Here's how the part is built. I have some questions about the finished solid (model axes, mm). Face numbers are marked on the shaded views. Round coordinates to 2 decimals unless told otherwise and drop trailing zeros. Order: outer loops, then holes, each group sorted by start corner. A loop starts at its lowest first (then second) coordinate and runs counter-clockwise, first axis right, second up.
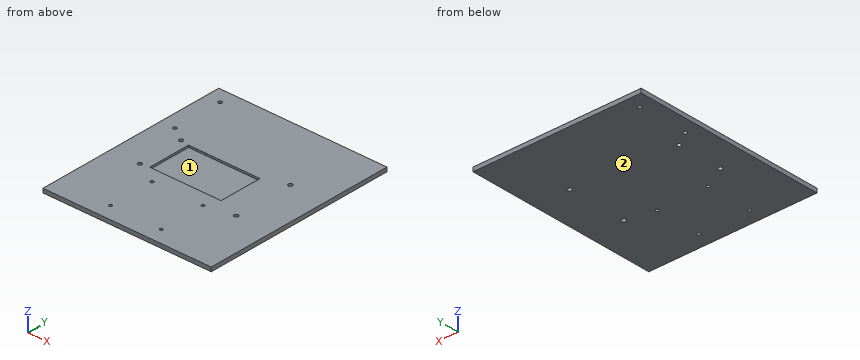
```python
from build123d import *

# Parameters (mm, degrees)
ESQUISSE1_W             = 165
ESQUISSE1_H             = 190
BOSS_EXTRU_1_DEPTH      = 4
ESQUISSE2_R             = 2
ENL_V_MAT_EXTRU_1_DEPTH = 10
ESQUISSE3_R             = 1.75
ENL_V_MAT_EXTRU_2_DEPTH = 10
ESQUISSE4_R             = 1.5
ENL_V_MAT_EXTRU_3_DEPTH = 10
ESQUISSE5_W             = 70
ESQUISSE5_H             = 42
ENL_V_MAT_EXTRU_4_DEPTH = 2


with BuildPart() as part:
    # Esquisse1 → Boss.-Extru.1 (new body)
    with BuildSketch(Plane.XY):
        with Locations((82.5, 95)):
            Rectangle(ESQUISSE1_W, ESQUISSE1_H)
    extrude(amount=BOSS_EXTRU_1_DEPTH)

    # Esquisse2 → Enlèv. mat.-Extru.1 (cut)
    with BuildSketch(Plane(origin=(0, 0, 0), x_dir=(-1, 0, 0), z_dir=(0, 0, -1))):
        with Locations((-129.934319196, 124.25)):
            Circle(ESQUISSE2_R)
        with Locations((-29, 117.25)):
            Circle(ESQUISSE2_R)
        with Locations((-29, 72.75)):
            Circle(ESQUISSE2_R)
        with Locations((-129.934319196, 65.75)):
            Circle(ESQUISSE2_R)
    extrude(amount=-ENL_V_MAT_EXTRU_1_DEPTH, mode=Mode.SUBTRACT)

    # Esquisse3 → Enlèv. mat.-Extru.2 (cut)
    with BuildSketch(Plane.XY.offset(4)):
        with Locations((14, 176)):
            Circle(ESQUISSE3_R)
        with Locations((14, 127)):
            Circle(ESQUISSE3_R)
    extrude(amount=-ENL_V_MAT_EXTRU_2_DEPTH, mode=Mode.SUBTRACT)

    # Esquisse4 → Enlèv. mat.-Extru.3 (cut)
    with BuildSketch(Plane.XY.offset(4)):
        with Locations((52.5, 15)):
            Circle(ESQUISSE4_R)
        with Locations((52.5, 60)):
            Circle(ESQUISSE4_R)
        with Locations((102.5, 60)):
            Circle(ESQUISSE4_R)
        with Locations((102.5, 15)):
            Circle(ESQUISSE4_R)
    extrude(amount=-ENL_V_MAT_EXTRU_3_DEPTH, mode=Mode.SUBTRACT)

    # Esquisse5 → Enlèv. mat.-Extru.4 (cut)
    with BuildSketch(Plane.XY.offset(4)):
        with Locations((72.5, 95)):
            Rectangle(ESQUISSE5_W, ESQUISSE5_H)
    extrude(amount=-ENL_V_MAT_EXTRU_4_DEPTH, mode=Mode.SUBTRACT)


solid = part.part
```
1. I need wall thicknesses on probe 1 along Y at (x, z) = (102.5, 1.4); probe 2 along Y at (x, z) = (47, 2.45); probe 3 along X at (y, z) = (81.5, 2.1). Which ranges of each line are inside material? Lowest first, please.
Evaluation:
probe 1: y = 0 to 13.5, 16.5 to 58.5, 61.5 to 190
probe 2: y = 0 to 74, 116 to 190
probe 3: x = 0 to 37.5, 107.5 to 165
2. If we section it at C-C, the plane y = 80: Write out the boundary of the cut face in (x, z).
Evaluation:
outline: (0, 0) - (165, 0) - (165, 4) - (107.5, 4) - (107.5, 2) - (37.5, 2) - (37.5, 4) - (0, 4) - close
3. If we section it at A-A, the plane z = 3.35: State how many separate pieces and enclosed holes the cut face has, and give its area (3 significant figures).
Evaluation:
separate pieces: 1
enclosed holes: 11
area: 28,300 mm2
4. I'm going to push flat-ended pins straight in: P1, Ø3, axis at x = 14, y = 127, coming from the -Z side; P2, Ø10, axis at x = 77, y = 106, coming from the -Z side; P3, Ø12.5, axis at x = 66, y = 91.5, coming from the +Z side. Where does each tip first touch, or does it pass through?
Evaluation:
P1: passes through
P2: stops at z = 0
P3: stops at z = 2
5. If we section it at B-B, the plane x = 74: Write out the boundary of the cut face in (y, z).
Evaluation:
outline: (0, 0) - (190, 0) - (190, 4) - (116, 4) - (116, 2) - (74, 2) - (74, 4) - (0, 4) - close
6. If we mould it in two halves opening along X, with no side actions, what happens to the marked faces 1 and 2? For each: released by +X, released by -X, zero draft, split by the parting line, or undercut.
Evaluation:
face 1: undercut
face 2: zero draft
